from build123d import *

# Parameters (mm, degrees)
F0_W      = 200
F0_H      = 13
F1_DEPTH  = 15
F2_R      = 8
F3_DEPTH  = 3
F4_R      = 8
F5_DEPTH  = 3
F6_R      = 4
F7_DEPTH  = 13
F8_R      = 8
F9_DEPTH  = 7
F11_DEPTH = 25
F12_R     = 4
F13_DEPTH = 25
F15_DEPTH = 25


with BuildPart() as f1:
    # F0 (on Top) → F1 (new body)
    with BuildSketch(Plane.XY):
        with Locations((69.0846356191, 17.0292752752)):
            Rectangle(F0_W, F0_H)
    extrude(amount=F1_DEPTH)

    # F2 (on face) → F3 (join)
    with BuildSketch(Plane.XZ.offset(-10.5292752752)):
        with Locations((-30.4153643809, 13.36)):
            Circle(F2_R)
    extrude(amount=-F3_DEPTH)

    # F4 (on face) → F5 (join)
    with BuildSketch(Plane(origin=(0, 23.5292752752, 0), x_dir=(-1, 0, 0), z_dir=(0, 1, 0))):
        with Locations((30.4153643809, 13.36)):
            Circle(F4_R)
    extrude(amount=-F5_DEPTH)

    # F6 (on face) → F7 (cut)
    with BuildSketch(Plane(origin=(0, 23.5292752752, 0), x_dir=(-1, 0, 0), z_dir=(0, 1, 0))):
        with Locations((30.4153643809, 13.36)):
            Circle(F6_R)
    extrude(amount=-F7_DEPTH, mode=Mode.SUBTRACT)

    # F8 (on face) → F9 (cut)
    with BuildSketch(Plane.XZ.offset(-20.5292752752)):
        with Locations((-30.4153643809, 13.36)):
            Circle(F8_R)
    extrude(amount=F9_DEPTH, mode=Mode.SUBTRACT)

    # F10 (on face) → F11 (cut)
    with BuildSketch(Plane.XZ.offset(-10.5292752752)):
        Polygon((169.0846356191, 15), (-22.5852685961, 15), (169.0846356191, 13), align=None)
    extrude(amount=-F11_DEPTH, mode=Mode.SUBTRACT)

    # F12 (on face) → F13 (cut)
    with BuildSketch(Plane.YZ.offset(169.0846356191)):
        with Locations((17.0292752752, 6.5)):
            Circle(F12_R)
    extrude(amount=-F13_DEPTH, mode=Mode.SUBTRACT)

    # F14 (on face) → F15 (cut)
    with BuildSketch(Plane(origin=(0, 23.5292752752, 0), x_dir=(-1, 0, 0), z_dir=(0, 1, 0))):
        Polygon((23.4402101487, 3.3569312654), (20.2043242753, 11.7502389476), (4.9986368977, 3.3569312654), align=None)
        Polygon((-8.0218771473, 3.0973160174), (8.4835188463, 10.455628857), (-8.0218771473, 10.7478844002), align=None)
        Polygon((-34.541686737, 3.0973160174), (-13.1043503061, 3.0973160174), (-13.1043503061, 11.0331652686), align=None)
        Polygon((-50.001192838, 3.2930115703), (-29.0924943984, 11.0331652686), (-50.001192838, 11.0331652686), align=None)
        Polygon((-83.6627408862, 3.0973160174), (-56.263808161, 3.0973160174), (-56.263808161, 10.7733560726), align=None)
        Polygon((-102.4060808122, 3.0973160174), (-75.007148087, 10.7733560726), (-102.4060808122, 10.7733560726), align=None)
        Polygon((-132.8051537275, 3.0973160174), (-108.0802679062, 3.0973160174), (-108.0802679062, 10.7733560726), align=None)
    extrude(amount=-F15_DEPTH, mode=Mode.SUBTRACT)


solid = f1.part
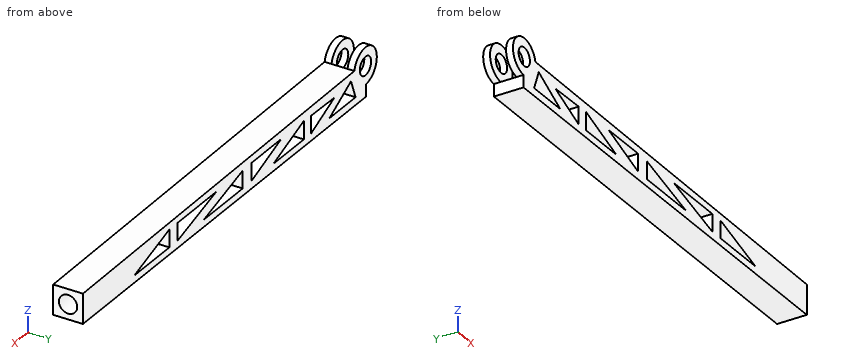
Part model, mm, in its own coordinate system. Coordinates: 2 decimals unless noted, no trailing zeros. Loops run counter-clockwise (first coordinate to the right, second up) from the corner with the lowest first, then second, coordinate; pieces in that order, holes last. Notation, with made-up numbers: (51.5, -8.5) - (75.5, -8.5) arc R5 ccw to (75.5, -0.5) - close; hole circle Ø5 at (69.25, -19). An arc over 180 degrees is marked (long way). Write each question's results on one line, items separated by ' | '. Start each with the question number.
Q1. Slice it at C-C on x = 19. Give the cut face in (y, z), and give its area (3 significant figures).
Q2. Probe line 1 along Y through (x, z) = (-26.5, 19.5); line 2 along X through (y, z) = (22.25, 2); line 3 along Z through (x, y) = (-7.5, 18.5). List the from-to ranges inside material, lowest first.
Q3. Slice it at A-A on x = 46. Give the cut face in (y, z).
Q4. Drop flat-ended pins along their axis: pin 1 Ø5 at (x, y) = (49, 20.5) entering from +Z; pin 2 Ø1 at (x, y) = (133.5, 19.5) entering from +Z; pin 3 Ø4 at (y, z) = (18, 7.5) entering from +X. Give the stop position or say it passes through.
Q5. Slice it at B-B on y = 17. Give the number of separate pieces and of enclosed holes in the cut face, and give its area (3 significant figures).
Answer:
1) outline: (10.53, 0) - (23.53, 0) - (23.53, 3.1) - (10.53, 3.1) - close; (10.53, 8.85) - (23.53, 8.85) - (23.53, 14.57) - (10.53, 14.57) - close | area: 115 mm2
2) line 1: y = 10.53 to 13.53, 20.53 to 23.53 | line 2: x = -30.92 to 169.08 | line 3: z = 0 to 3.36, 4.74 to 10.02, 10.47 to 14.84
3) outline: (10.53, 0) - (23.53, 0) - (23.53, 4.77) - (10.53, 4.77) - close; (10.53, 11.03) - (23.53, 11.03) - (23.53, 14.28) - (10.53, 14.28) - close
4) pin 1: stops at z = 14.28 | pin 2: stops at z = 13.38 | pin 3: stops at x = 144.08
5) separate pieces: 1 | enclosed holes: 7 | area: 1,930 mm2
